Study the drawing (mm; zero at the part's minimum x, y, z) and answer. A direction names the side the tool comes from. Coordinates: 2 decimals unless noted, no trailing zeros. Write each loop counter-clockwise with the first axis right and the second up, starting at its lowest first coordinate (ties: lowest second). Pieces come first, ordered by that corner, then holes. Notation, with made-up numbers: (59, 81.25) -> (75, 81.25) arc R23 ccw to (75, 90.25) -> close; hole circle Ø2 at (31.25, 15). An arc over 180 degrees is marked (long way). Answer in a Markdown table with one row per item. Add a question column.
Item 1: Section A-A on z = 460 is taken. Write down the section's boundary in (x, y).
Item 2: Section D-D on z = 812.5 is taken. Write down the section's boundary in (x, y) (1 decimal), then the cut area to 3 significant figures.
Item 3: Section C-C on y = 545.5 is taken. Write down the section's boundary in (x, z).
Item 4: Section B-B on x = 1299 is taken. Write down the section's boundary in (y, z), then the cut area to 3 significant figures.
Item 5: Straight lines are drawn through the part: line 1 (X direction, y = 268, z = 264.5); line 2 (Z direction, x = 1040.5, y = 972); line 3 (Y direction, x = 1595.5, z = 577). For each, find the intervals that lie inside material, in ascending order. Write a range as from..to.
Item 6: Given pin 1 Ø8 at (y, z) = (975.5, 107.5) entering from +X (1 decimal); pin 2 Ø1 at (y, z) = (653.5, 325) entering from +X; pin 3 Ø10 at (x, z) = (935, 703) entering from +Y, each flat-ended and moving along its own axis, determine where each tip first touches the part or whether it passes through.
Item 7: Which of the six approach directions +Z, -Z, +X, -X, +Y, -Y give full straight-line access (tool end or side, diameter ignored) to the marked faces 1, 2, 3, 4 and 5?
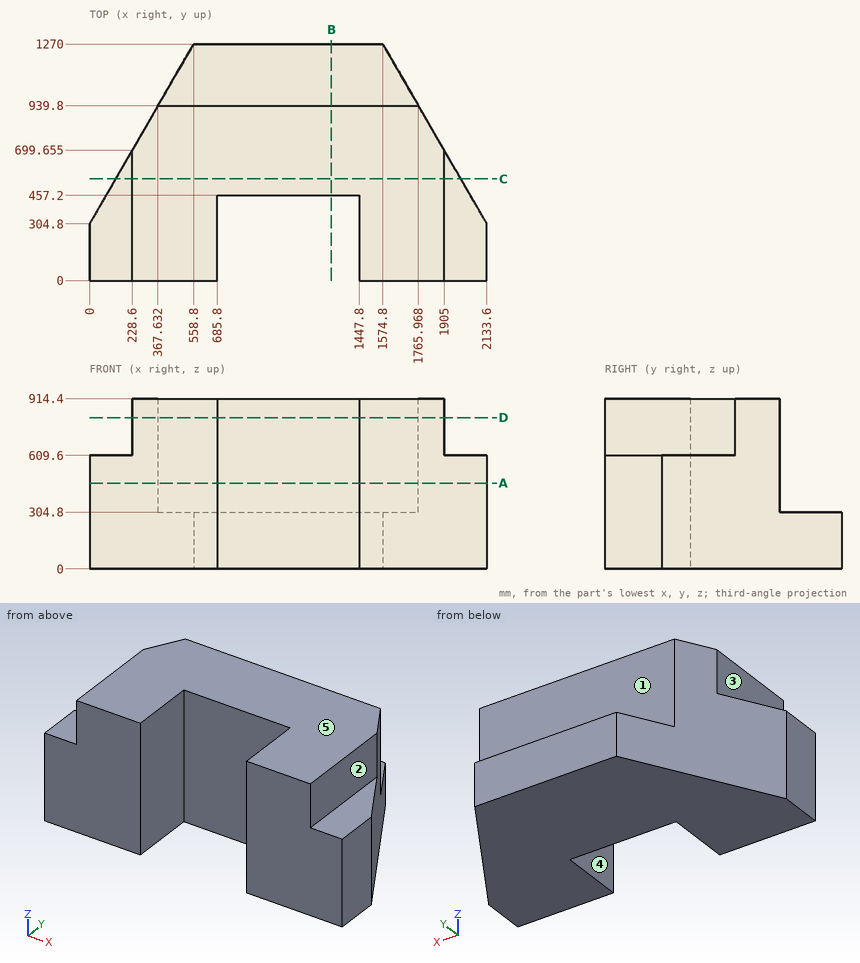
Results below:
| question | item | result |
|---|---|---|
| 1 | outline | (0, 0) -> (685.8, 0) -> (685.8, 457.2) -> (1447.8, 457.2) -> (1447.8, 0) -> (2133.6, 0) -> (2133.6, 304.8) -> (1765.97, 939.8) -> (367.63, 939.8) -> (0, 304.8) -> close |
| 2 | outline | (228.6, 0) -> (685.8, 0) -> (685.8, 457.2) -> (1447.8, 457.2) -> (1447.8, 0) -> (1905, 0) -> (1905, 699.7) -> (1766, 939.8) -> (367.6, 939.8) -> (228.6, 699.7) -> close |
| 2 | area | 1,190,000 mm2 |
| 3 | outline | (139.35, 0) -> (1994.25, 0) -> (1994.25, 609.6) -> (1905, 609.6) -> (1905, 914.4) -> (228.6, 914.4) -> (228.6, 609.6) -> (139.35, 609.6) -> close |
| 4 | outline | (457.2, 0) -> (1270, 0) -> (1270, 304.8) -> (939.8, 304.8) -> (939.8, 914.4) -> (457.2, 914.4) -> close |
| 4 | area | 542,000 mm2 |
| 5 | line 1 | x = 0..685.8, 1447.8..2133.6 |
| 5 | line 2 | z = 0..304.8 |
| 5 | line 3 | y = 0..939.8 |
| 6 | pin 1 | stops at x = 1747.6 |
| 6 | pin 2 | stops at x = 1932.01 |
| 6 | pin 3 | stops at y = 939.8 |
| 7 | face 1 | +Z, +X, -X, +Y |
| 7 | face 2 | +Z, +X, +Y, -Y |
| 7 | face 3 | +Z, -X, +Y, -Y |
| 7 | face 4 | +Z, -Z, -Y |
| 7 | face 5 | +Z, +X, -X, +Y, -Y |
